from build123d import *

# Parameters (mm, degrees)
BASE_ROUE_DEPTH         = 15
ESQUISSE2_R             = 19.5
VIDE_ROUE_DEPTH         = 13
ESQUISSE3_R             = 4.5
AXE_ROUE_DEPTH          = 5
ESQUISSE4_R             = 18
ROUE_DEPTH              = 11
ESQUISSE6_R             = 5
VIS_DEPTH               = 32
ENL_V_START             = -18
ESQUISSE7_R             = 5
ESQUISSE7_R_2           = 3
ENL_V_MAT_EXTRU_3_DEPTH = 18


with BuildPart() as part:
    # Esquisse1 → BASE ROUE (new body)
    with BuildSketch(Plane(origin=(0, 0, 0), x_dir=(0, 0, -1), z_dir=(1, 0, 0))):
        with BuildLine():
            Line((-18.33030278, -8), (18.33030278, -8))
            ThreePointArc((18.33030278, -8), (0, 20), (-18.33030278, -8))
        make_face()
    base_roue = extrude(amount=BASE_ROUE_DEPTH)

    # Esquisse2 → VIDE ROUE (cut)
    with BuildSketch(Plane(origin=(15, 0, 0), x_dir=(0, 0, -1), z_dir=(1, 0, 0))):
        Circle(ESQUISSE2_R)
    vide_roue = extrude(amount=-VIDE_ROUE_DEPTH, mode=Mode.SUBTRACT)

    # Esquisse3 → AXE ROUE (add)
    with BuildSketch(Plane(origin=(2, 0, 0), x_dir=(0, 0, -1), z_dir=(1, 0, 0))):
        Circle(ESQUISSE3_R)
    axe_roue = extrude(amount=AXE_ROUE_DEPTH)

    # Esquisse4 → ROUE (add)
    with BuildSketch(Plane(origin=(7, 0, 0), x_dir=(0, 0, -1), z_dir=(1, 0, 0))):
        Circle(ESQUISSE4_R)
    roue = extrude(amount=ROUE_DEPTH)

    # SYM ROUE + BASE: BASE ROUE, VIDE ROUE, AXE ROUE, ROUE across plane
    add(base_roue.mirror(Plane(origin=(0, 0, 0), x_dir=(0, 0, 1), z_dir=(1, 0, 0))))
    add(vide_roue.mirror(Plane(origin=(0, 0, 0), x_dir=(0, 0, 1), z_dir=(1, 0, 0))), mode=Mode.SUBTRACT)
    add(axe_roue.mirror(Plane(origin=(0, 0, 0), x_dir=(0, 0, 1), z_dir=(1, 0, 0))))
    add(roue.mirror(Plane(origin=(0, 0, 0), x_dir=(0, 0, 1), z_dir=(1, 0, 0))))

    # Esquisse6 → VIS (add)
    with BuildSketch(Plane(origin=(0, 5, 0), x_dir=(1, 0, 0), z_dir=(0, 1, 0))):
        with Locations(Location((0, 14, 0), (0, 0, 90))):
            Circle(ESQUISSE6_R)
    extrude(amount=VIS_DEPTH)

    # Esquisse7 → Enlèv. mat.-Extru.3 (cut)
    with BuildSketch(Plane(origin=(0, 37, 0), x_dir=(1, 0, 0), z_dir=(0, 1, 0)).offset(ENL_V_START)):
        with Locations(Location((0, 14, 0), (0, 0, 90))):
            Circle(ESQUISSE7_R)
        with Locations(Location((0, 14, 0), (0, 0, 270))):
            Circle(ESQUISSE7_R_2, mode=Mode.SUBTRACT)
    extrude(amount=ENL_V_MAT_EXTRU_3_DEPTH, mode=Mode.SUBTRACT)


solid = part.part
Read the model definition and answer for the solid it produces. Units are mm, in the model's axes. A direction names the side the tool comes from. Give positions to 0.01 mm unless a question says otherwise; leave off trailing zeros. Write each loop counter-clockwise with the first axis right and the second up, starting at its lowest first coordinate (ties: lowest second). Pieces come first, ordered by that corner, then holes. Notation, with made-up numbers: M 67,88.5 L 85,88.5 A16 cw 85,100.5 Z; hole C 82,9 d5. An arc over 180 degrees is marked long. One line per item, written item: value. Start each with the question number.
(1) A tool of negligible diameter and unlimited length cuts with its end or side. For faces 4 (the cylindrical face through (0, 28, -17)), 5 (the flat face through (-2, 6, 0)), 6 (the cylindrical face through (-12.423, 17.847, 2.343)), 7 (the cylindrical face through (8.591, 19.492, -0.544)), from which of +Z, -Z, +X, -X, +Y, -Y can it reach the whole face along a straight path? Write none if from no direction.
(2) Find section A-A (y = 0). Determine the outline of the cut face in (x, z).
(3) Flat-ended cylindrical pins translate along their axes: pin 1 Ø10 at (x, y) = (-5, 18.5) entering from +Z; pin 2 Ø15 at (x, z) = (4.5, 8.5) entering from -Y; pin 3 Ø1.5 at (x, z) = (-3, -14) entering from -Y. Find the tip coordinate at first contact, or state that the pin passes through.
(4) Find the intervals of material crossed by line 1 (X direction, y = 16, z = -2); line 2 (Y direction, x = 12, z = 0); line 3 (X direction, y = -11.5, z = -7), in increasing order.
(5) Find section B-B (y = -12.5). Determine the outline of the cut face in (x, z).
(6) Determine the mould class of faces 1 (the flat face through (15, 19.5, 3.1)), 2 (the cylindrical face through (12.423, 17.847, 2.343)), 3 (the flat face through (0, -8, 0)) for opening direction Y: pulls with the +Y half, pulls with the -Y half, needs draft (parallel to the pull), parting line crosses it, or undercut.
(7) Find section C-C (z = 16). Determine the outline of the cut face in (x, y).
(8) Find section D-D (x = 12). Determine the outline of the cut face in (y, z), plus the area to 3 significant figures.
Results below:
1. face 4: +Y
1. face 5: none
1. face 6: -X
1. face 7: +X
2. outline: M -18,-18 L -7,-18 L -7,-4.5 L -2,-4.5 L -2,-19.5 L -15,-19.5 L -15,-20 L 15,-20 L 15,-19.5 L 2,-19.5 L 2,-4.5 L 7,-4.5 L 7,-18 L 18,-18 L 18,18 L 7,18 L 7,4.5 L 2,4.5 L 2,19.5 L 15,19.5 L 15,20 L -15,20 L -15,19.5 L -2,19.5 L -2,4.5 L -7,4.5 L -7,18 L -18,18 Z
3. pin 1: stops at z = 14.76
3. pin 2: stops at y = -17.94
3. pin 3: stops at y = 5
4. line 1: x = -18 to -7, -2 to 2, 7 to 18
4. line 2: y = -18 to 18, 19.5 to 20
4. line 3: x = -18 to -7, 7 to 18
5. outline: M -18,-12.95 L -7,-12.95 L -7,12.95 L -18,12.95 Z; M 7,-12.95 L 18,-12.95 L 18,12.95 L 7,12.95 Z
6. face 1: needs draft
6. face 2: undercut
6. face 3: pulls with the -Y half
7. outline: M -18,-8.25 L -7,-8.25 L -7,8.25 L -18,8.25 Z; M -15,11.15 L -2,11.15 L -2,-8 L 2,-8 L 2,11.15 L 15,11.15 L 15,12 L -15,12 Z; M 7,-8.25 L 18,-8.25 L 18,8.25 L 7,8.25 Z
8. outline: C 0,0 d36; M -8,-18.33 A20 ccw long -8,18.33 L -8,17.78 A19.5 cw long -8,-17.78 Z
8. area: 1,060 mm^2
